The figure shows three views and two pictorial views of one solid part (mm, origin at its lowest corner). Answer the questions. A direction names the side the tool comes from. Round coordinates to 2 decimals unless told otherwise and drop trailing zeros. Loops run counter-clockwise (first coordinate to the right, second up) from the corner with the lowest first, then second, coordinate; pieces in that order, holes last. Notation, with made-up numbers: (78, 34.5) -> (129, 34.5) arc R7 ccw to (129, 44.5) -> close; hole circle Ø6 at (-14.75, 18). An arc over 180 degrees is marked (long way). Put each result on its own line as item: value.
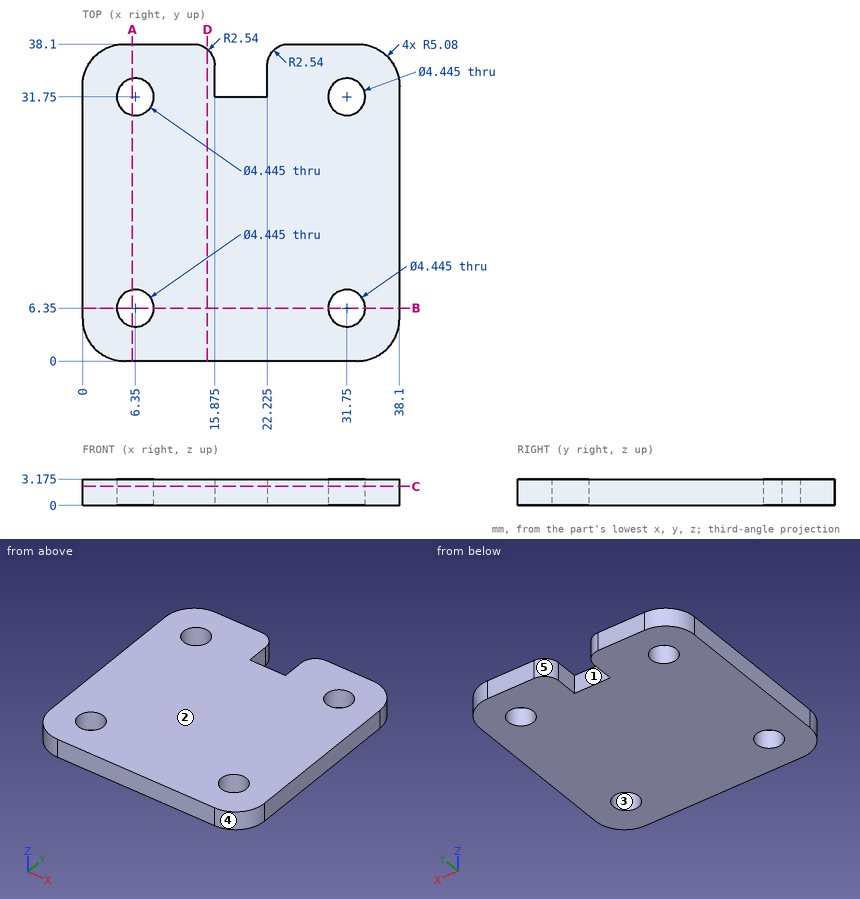
Item 1: The part is cut by section B-B (y = 6.35). Determine the outline of the cut face in (x, z) (1 decimal), then the cut area to 3 significant figures.
Derived:
outline: (0, 0) -> (4.1, 0) -> (4.1, 3.2) -> (0, 3.2) -> close; (8.6, 0) -> (29.5, 0) -> (29.5, 3.2) -> (8.6, 3.2) -> close; (34, 0) -> (38.1, 0) -> (38.1, 3.2) -> (34, 3.2) -> close
area: 92.7 mm^2
Item 2: A flat-ended cylindrical pin translates along its axis: pin 1 Ø4 at (x, y) = (31.75, 31.75) entering from -Z. Find the tip coordinate at first contact, or state that the pin passes through.
Derived:
pin 1: passes through
Item 3: The part is cut by section C-C (z = 2.3). State how many separate pieces and enclosed holes the cut face has, then the cut area to 3 significant figures.
Derived:
separate pieces: 1
enclosed holes: 4
area: 1,320 mm^2
Item 4: The part is cut by section D-D (x = 15). Determine the outline of the cut face in (y, z) (3 decimals), then the cut area to 3 significant figures.
Derived:
outline: (0, 0) -> (37.478, 0) -> (37.478, 3.175) -> (0, 3.175) -> close
area: 119 mm^2
Item 5: The part is cut by section A-A (x = 6). Determine the outline of the cut face in (y, z) (3 decimals).
Derived:
outline: (0, 0) -> (4.155, 0) -> (4.155, 3.175) -> (0, 3.175) -> close; (8.545, 0) -> (29.555, 0) -> (29.555, 3.175) -> (8.545, 3.175) -> close; (33.945, 0) -> (38.1, 0) -> (38.1, 3.175) -> (33.945, 3.175) -> close
Item 6: Find the intervals of material crossed by line 1 along X through (y, z) = (8, 2.5); line 2 along X through (y, z) = (32, 2.1) (3 decimals); line 3 along Y through (x, z) = (16.5, 0.85), in increasing order.
Derived:
line 1: x = 0 to 4.86, 7.84 to 30.26, 33.24 to 38.1
line 2: x = 0 to 4.142, 8.558 to 15.875, 22.225 to 29.542, 33.958 to 38.1
line 3: y = 0 to 31.75
Item 7: For a pull along Y with two mould halves and no side action, classify the marked faces 3, 4 and 5 as pulls with the +Y half, pulls with the -Y half, needs draft (parallel to the pull), parting line crosses it, or undercut.
Derived:
face 3: undercut
face 4: pulls with the -Y half
face 5: pulls with the +Y half
Item 8: Which of the six approach directions +Z, -Z, +X, -X, +Y, -Y give full straight-line access (tool end or side, diameter ignored) to the marked faces 1 and 2?
Derived:
face 1: +Z, -Z, +Y
face 2: +Z, +X, -X, +Y, -Y
